Part print with two shaded views. Sizes in mm from the minimum x, y, z corner. A direction names the side the tool comes from. Coordinates: 2 decimals unless noted, no trailing zeros. Order: outer loops, then holes, each group sorted by start corner. A loop starts at its lowest first (then second) coordinate and runs counter-clockwise, first axis right, second up. Notation, with made-up numbers: (19.25, 35) - (66.25, 35) arc R14 ccw to (66.25, 40) - close; hole circle Ø8 at (-35, 57.5). An arc over 180 degrees is marked (long way). Return JSON: item names as keys, results as strings.
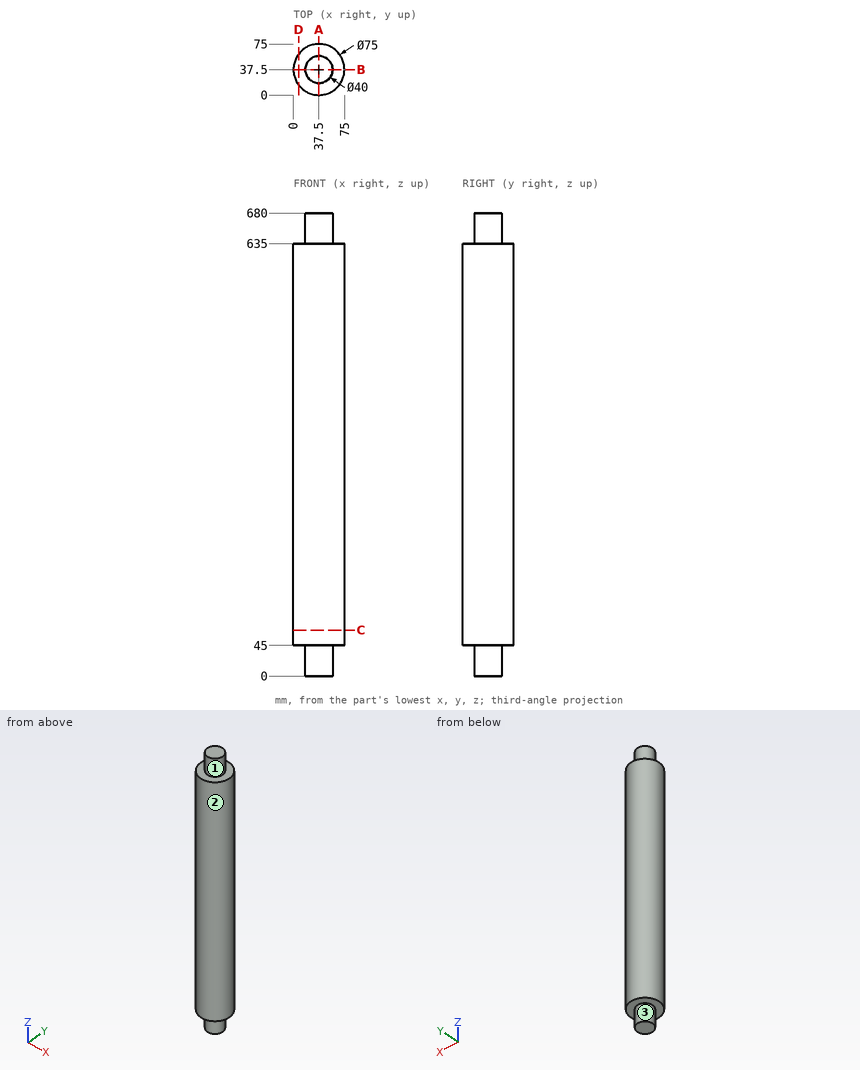
Item 1: Wall check: L1, parallel to Z at x = 28, y = 11; L2, parallel to Y at x = 4, z = 235.5; L3, parallel to Y at x = 66.5, z = 599.5. Give the ranges that are in metal, low to high. Write a range as [from, to].
Findings below:
{"L1": "z = [45, 635]", "L2": "y = [20.65, 54.35]", "L3": "y = [13.73, 61.27]"}
Item 2: Band-saw the part on A-A, the plane x = 37.5. List the corners of the cut face in (y, z).
Findings below:
{"outline": "(0, 45) - (17.5, 45) - (17.5, 0) - (57.5, 0) - (57.5, 45) - (75, 45) - (75, 635) - (57.5, 635) - (57.5, 680) - (17.5, 680) - (17.5, 635) - (0, 635) - close"}
Item 3: Which spindle directions (+Z, -Z, +X, -X, +Y, -Y) get a long thin tool onto all of the face, cutting with end or side? Do the marked faces 1, 2 and 3. Say none if no direction does.
Findings below:
{"face 1": "+Z", "face 2": "+Z, -Z", "face 3": "-Z"}
Item 4: Band-saw the part on D-D, the plane x = 7.5. List the corners of the cut face in (y, z), then the cut area to 4 significant figures.
Findings below:
{"outline": "(15, 45) - (60, 45) - (60, 635) - (15, 635) - close", "area": "26,550 mm²"}
Item 5: Band-saw the part on C-C, the plane z = 67.5. List the corners of the cut face in (x, y).
Findings below:
{"outline": "circle Ø75 at (37.5, 37.5)"}
Item 6: Drop flat-ended pins along their axis: P1, Ø2, axis at y = 50.5, z = 502.5, coming from the -X side; P2, Ø8, axis at y = 63.5, z = 169.5, coming from the -X side; P3, Ø5, axis at x = 26, z = 406.5, coming from the -Y side. Give the stop position or say it passes through.
Findings below:
{"P1": "stops at x = 1.97", "P2": "stops at x = 7.13", "P3": "stops at y = 1.1"}
